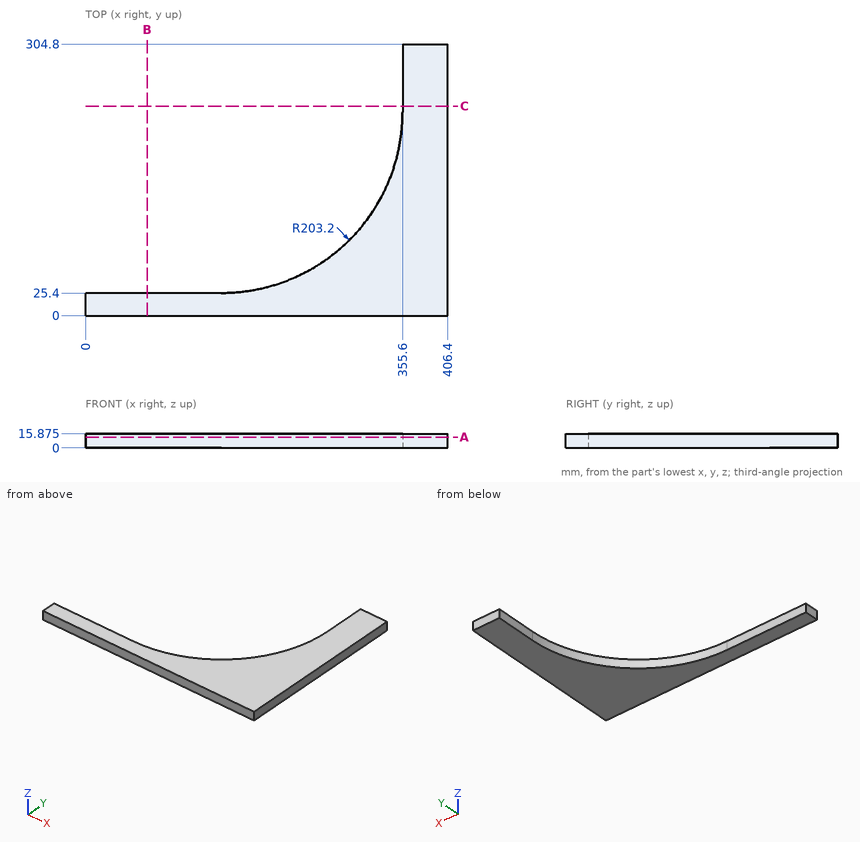
Geometry check sheet. Reference: drawing and pictorial views, mm from the part's lowest x, y, z. Round coordinates to 2 decimals unless told otherwise and drop trailing zeros. Loops run counter-clockwise (first coordinate to the right, second up) from the corner with the lowest first, then second, coordinate; pieces in that order, holes last. Notation, with made-up numbers: M -28.75,73.25 L -15.75,73.25 A25 ccw -15.75,107.25 Z; hole C 29,34 d11. An arc over 180 degrees is marked long. Return JSON: item names as keys, results as strings. Group by question number.
(1) Section check A-A, the plane z = 12. Enter the section's corners in (x, y), and give its area (3 significant figures).
(2) Go/stop test with flat-tipped pins: pin 1 (8 mm diameter, centred on x = 107.5, z = 5, fed in from +Y); pin 2 (8 mm diameter, centred on y = 278, z = 6, fed in from -X); pin 3 (4 mm diameter, centred on y = 158.5, z = 13.5, fed in from -X). Record where each tip stops, or that it passes through.
(3) Section check B-B, the plane x = 69. Enter the section's corners in (y, z) (3 decimals), and give its area (3 significant figures).
(4) Section check C-C, the plane y = 235. Enter the section's corners in (x, z) (3 decimals), and give its area (3 significant figures).
(5) Scan lines: line 1 along Y through (x, z) = (108, 14); line 2 along X through (y, z) = (281.5, 12.5); line 3 along X through (y, z) = (98, 7.75). Record each from-to range of solid material in increasing order. Write a range as [from, to].
Data:
{
 "1": {"outline": "M 0,0 L 406.4,0 L 406.4,304.8 L 355.6,304.8 L 355.6,228.6 A203.2 cw 152.4,25.4 L 0,25.4 Z", "area": "33,400 mm²"},
 "2": {"pin 1": "y = 25.4", "pin 2": "x = 355.6", "pin 3": "x = 342.38"},
 "3": {"outline": "M 0,0 L 25.4,0 L 25.4,15.875 L 0,15.875 Z", "area": "403 mm²"},
 "4": {"outline": "M 355.6,0 L 406.4,0 L 406.4,15.875 L 355.6,15.875 Z", "area": "806 mm²"},
 "5": {"line 1": "[0, 25.4]", "line 2": "[355.6, 406.4]", "line 3": "[308.07, 406.4]"}
}
